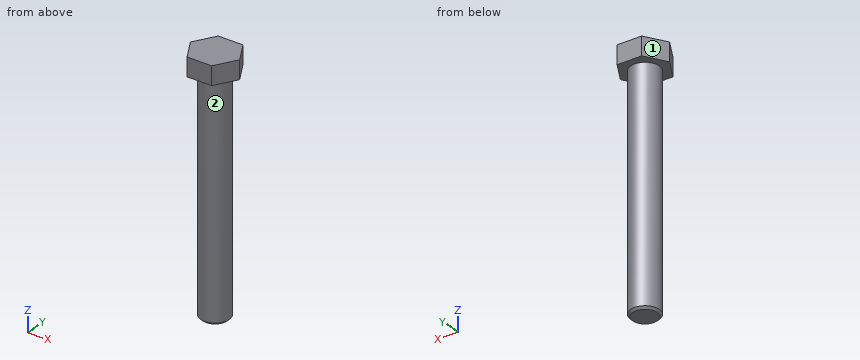
Solid Edge part; units mm, degrees
sketch "Sketch1" plane through (0, 0, 0) normal (0, 0, 1) x (1, 0, 0)
  circle A0 centre (0, 0) radius 11.049
extrude "Protrusion1" add sketch "Sketch1" along normal blind 8.2042
sketch "Sketch2" plane through (0, 0, 0) normal (0, 0, -1) x (1, 0, 0)
  circle A0 centre (0, 0) radius 6.35
extrude "Protrusion2" add sketch "Sketch2" along normal blind 101.6
sketch "Sketch3" plane through (0, 0, -101.6) normal (0, 0, -1) x (1, 0, 0)
  circle A0 centre (0, 0) radius 6.3497
extrude "Cutout1" cut sketch "Sketch3" against normal blind 101.473 flip side to cut
chamfer "Chamfer_1" distance 0.9525 angle 45 1 edges at (-6.3497, 0, -101.6)
sketch "Sketch4" plane through (0, 0, 8.2042) normal (0, 0, 1) x (1, 0, 0)
  line L0 (-5.5995, 9.525) -> (5.5995, 9.525)
extrude "Cutout2" cut sketch "Sketch4" against normal up to next material side at (0, 9.575, 8.2042)
pattern_circular "Pattern1" count 6 over 360 about axis through (0, 0, 8.2042) along (0, 0, 1) of "Cutout2"
properties part number "159699"
Work out the finished part from the listing and answer in its coordinate system (mm). Face numbers are marked on the shaded views. A direction names the side the tool comes from. Round coordinates to 2 decimals unless told otherwise and drop trailing zeros. Loops run counter-clockwise (first coordinate to the right, second up) from the corner with the lowest first, then second, coordinate; pieces in that order, holes last. Notation, with made-up numbers: (-24, 73.5) -> (17, 73.5) arc R23 cw to (17, 86.5) -> close; hole circle Ø1 at (86.25, 82). An arc over 180 degrees is marked (long way). Write each question's results on one line, items separated by ' | '. Start each with the question number.
1. A tool of negligible diameter and unlimited length cuts with its end or side. For the marked faces 1 and 2, from which of +Z, -Z, +X, -X, +Y, -Y can it reach the whole face along a straight path? Write none if from no direction.
2. Section C-C (x = -8.5) is taken. Determine the outline of the cut face in (y, z), plus the area to 3 significant figures.
3. Given pin 1 Ø1.5 at (x, z) = (-6, -5.5) entering from -Y; pin 2 Ø1 at (x, z) = (2, -30) entering from +Y; pin 3 Ø2 at (y, z) = (-6.5, -62) entering from +X, each flat-ended and moving along its own axis, determine where each tip first touches the part or whether it passes through.
4. Find the intervals of material crossed by probe 1 along Z at (x, y) = (-7.5, -5.5); probe 2 along Y at (x, z) = (-4, -28); probe 3 along Y at (x, z) = (-4.5, -38), in increasing order. Write a range as from..to.
5. Section B-B (z = -77) is taken. Determine the outline of the cut face in (x, y), plus the area to 3 significant figures.
Evaluation:
1) face 1: +Z, -Z, -X, +Y | face 2: -Z
2) outline: (-4.33, 0) -> (4.33, 0) -> (4.33, 8.2) -> (-4.33, 8.2) -> close | area: 71.0 mm2
3) pin 1: stops at y = -3.57 | pin 2: stops at y = 6.17 | pin 3: stops at x = 3.17
4) probe 1: z = 0..8.2 | probe 2: y = -4.93..4.93 | probe 3: y = -4.48..4.48
5) outline: circle Ø12.7 at (0, 0) | area: 127 mm2
